Could you check a few things on this model? Use its own coordinates, in mm. Face numbers are marked on the shaded views. A direction names the side the tool comes from. Round coordinates to 2 decimals unless told otherwise and drop trailing zeros. Write each loop counter-clockwise with the first axis right and the second up, starting at its lowest first coordinate (ties: lowest second). Pieces come first, ordered by that corner, then holes. Notation, with made-up numbers: (56, 56) -> (75, 56) arc R18 ccw to (75, 74) -> close; hole circle Ø5 at (-4, 16). An arc over 180 degrees is marked (long way). Answer in a Markdown table with one row per item.
from build123d import *

# Parameters (mm, degrees)
F1_W     = 35
F1_H     = 25.5
F1_R     = 1
F1_W_2   = 24.5
F1_H_2   = 12.8
F1_R_2   = 2.05
F2_DEPTH = 3
F3_R     = 3
F4_R     = 1


with BuildPart() as f2:
    # F1 (on Top) → F2 (new body)
    with BuildSketch(Plane.XY):
        Rectangle(F1_W, F1_H)
        with Locations((-13.7, -2.55)):
            Circle(F1_R, mode=Mode.SUBTRACT)
        with Locations((0.35, -2.55)):
            Rectangle(F1_W_2, F1_H_2, mode=Mode.SUBTRACT)
        with Locations((14.3, -2.55)):
            Circle(F1_R, mode=Mode.SUBTRACT)
        with Locations((-11.5, 8.25)):
            Circle(F1_R_2, mode=Mode.SUBTRACT)
        with Locations((-3.5, 8.25)):
            Circle(F1_R_2, mode=Mode.SUBTRACT)
        with Locations((4.5, 8.25)):
            Circle(F1_R_2, mode=Mode.SUBTRACT)
        with Locations((12.5, 8.25)):
            Circle(F1_R_2, mode=Mode.SUBTRACT)
    extrude(amount=F2_DEPTH)

    # F3
    f3_edges = [f2.edges().sort_by_distance(p)[0] for p in [
        (-17.5, 12.75, 1.5),
        (17.5, 12.75, 1.5),
        (17.5, -12.75, 1.5),
        (-17.5, -12.75, 1.5),
    ]]
    fillet(f3_edges, radius=F3_R)

    # F4
    f4_edges = [f2.edges().sort_by_distance(p)[0] for p in [
        (-11.9, 3.85, 1.5),
        (12.6, 3.85, 1.5),
        (12.6, -8.95, 1.5),
        (-11.9, -8.95, 1.5),
    ]]
    fillet(f4_edges, radius=F4_R)


solid = f2.part
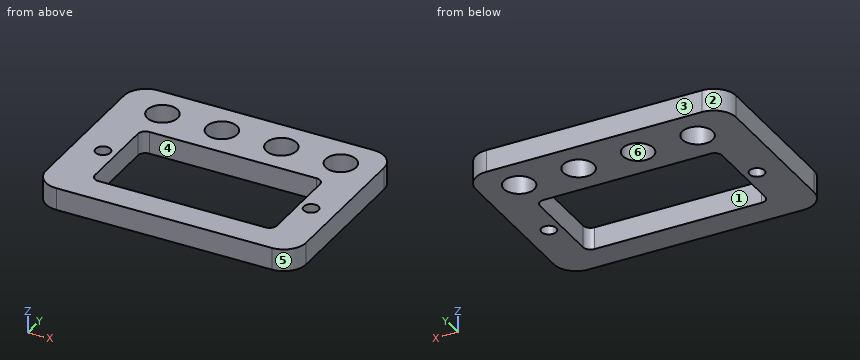
1) For pin 1 (1 mm diameter, centred on x = 2, y = 9.5, fed in from -Z), with a flat end and sliding along its axis, tell me the tip position at first contact or that it passes through.
Findings:
| item | result |
|---|---|
| pin 1 | stops at z = 0 |
2) Thinking about a two-plate mould opening in X: for the marked faces 3, 4, 5 and 6, which applies, +X half, -X half, draft (parallel to the pull), parting line (faces both ways), or undercut?
Findings:
| item | result |
|---|---|
| face 3 | draft |
| face 4 | undercut |
| face 5 | +X half |
| face 6 | undercut |
3) Imagine slicing it at B-B, the plane y = 8.25. Please give me the cut outline in (x, z), plus the area to 3 significant figures.
Findings:
| item | result |
|---|---|
| outline | (-17.5, 0) -> (-13.55, 0) -> (-13.55, 3) -> (-17.5, 3) -> close; (-9.45, 0) -> (-5.55, 0) -> (-5.55, 3) -> (-9.45, 3) -> close; (-1.45, 0) -> (2.45, 0) -> (2.45, 3) -> (-1.45, 3) -> close; (6.55, 0) -> (10.45, 0) -> (10.45, 3) -> (6.55, 3) -> close; (14.55, 0) -> (17.5, 0) -> (17.5, 3) -> (14.55, 3) -> close |
| area | 55.8 mm^2 |
4) Imagine slicing it at D-D, the plane y = -6. Please give me the cut outline in (x, z).
Findings:
| item | result |
|---|---|
| outline | (-17.5, 0) -> (-11.9, 0) -> (-11.9, 3) -> (-17.5, 3) -> close; (12.6, 0) -> (17.5, 0) -> (17.5, 3) -> (12.6, 3) -> close |
5) Imagine slicing it at A-A, the plane x = -11.5. Please give me the cut outline in (y, z).
Findings:
| item | result |
|---|---|
| outline | (-12.75, 0) -> (-8.75, 0) -> (-8.75, 3) -> (-12.75, 3) -> close; (3.65, 0) -> (6.2, 0) -> (6.2, 3) -> (3.65, 3) -> close; (10.3, 0) -> (12.75, 0) -> (12.75, 3) -> (10.3, 3) -> close |
6) Please list where these lines run through material, in increasing order: line 1 (Y direction, x = 4.5, z = 1.85); line 2 (Y direction, x = -13.7, z = 2.2); line 3 (X direction, y = -0.25, z = 1.8).
Findings:
| item | result |
|---|---|
| line 1 | y = -12.75 to -8.95, 3.85 to 6.2, 10.3 to 12.75 |
| line 2 | y = -12.75 to -3.55, -1.55 to 12.75 |
| line 3 | x = -17.5 to -11.9, 12.6 to 17.5 |
7) Imagine slicing it at C-C, the plane x = 1. Please give me the cut outline in (y, z).
Findings:
| item | result |
|---|---|
| outline | (-12.75, 0) -> (-8.95, 0) -> (-8.95, 3) -> (-12.75, 3) -> close; (3.85, 0) -> (12.75, 0) -> (12.75, 3) -> (3.85, 3) -> close |
8) For the marked faces 1 and 2, which set-ups out of +Z, -Z, +X, -X, +Y, -Y let a thin tool reach every point of the face, with its end or its side?
Findings:
| item | result |
|---|---|
| face 1 | +Z, -Z |
| face 2 | +Z, -Z, -X, +Y |
